from build123d import *

# Parameters (mm, degrees)
SKETCH1_W           = 20
SKETCH1_H           = 15
SKETCH1_W_2         = 15.2
SKETCH1_H_2         = 10.7
BOSS_EXTRUDE1_DEPTH = 21
SKETCH2_W           = 20
SKETCH2_H           = 15
SKETCH2_W_2         = 6.666666666
SKETCH2_H_2         = 5
BOSS_EXTRUDE2_DEPTH = 2
HOLE1_START         = -7.5
HOLE1_OUTLINE_R     = 1.25
HOLE1_DEPTH         = 15
FILLET1_R           = 1
SKETCH4_W           = 7
SKETCH4_H           = 3
CUT_EXTRUDE1_DEPTH  = 28.676705006


# Read off the part's stored shape, not the designer's step: Hole1
with BuildPart() as part:
    # Sketch1 → Boss-Extrude1 (new body)
    with BuildSketch(Plane(origin=(0, 0, 0), x_dir=(1, 0, 0), z_dir=(0, 1, 0))):
        Rectangle(SKETCH1_W, SKETCH1_H)
        Rectangle(SKETCH1_W_2, SKETCH1_H_2, mode=Mode.SUBTRACT)
    extrude(amount=BOSS_EXTRUDE1_DEPTH)

    # Sketch2 → Boss-Extrude2 (add)
    with BuildSketch(Plane.XZ):
        Rectangle(SKETCH2_W, SKETCH2_H)
        Rectangle(SKETCH2_W_2, SKETCH2_H_2, mode=Mode.SUBTRACT)
    extrude(amount=BOSS_EXTRUDE2_DEPTH)

    # Hole1 outline → Hole1 (cut)
    with BuildSketch(Plane.XY.offset(HOLE1_START)):
        with Locations((5.8, 3)):
            Circle(HOLE1_OUTLINE_R)
        with Locations((-5.8, 3)):
            Circle(HOLE1_OUTLINE_R)
    extrude(amount=HOLE1_DEPTH, mode=Mode.SUBTRACT)

    # Fillet1
    fillet1_edges = [part.edges().sort_by_distance(p)[0] for p in [
        (-10, 21, 0),
        (7.6, 21, 0),
        (0, 21, 7.5),
        (0, 21, -5.35),
        (-7.6, 21, 0),
        (0, 21, 5.35),
        (10, 21, 0),
        (10, 9.5, 7.5),
        (-10, 9.5, 7.5),
        (-10, 9.5, -7.5),
        (10, 9.5, -7.5),
        (0, 21, -7.5),
    ]]
    fillet(fillet1_edges, radius=FILLET1_R)

    # Sketch4 → Cut-Extrude1 (cut, through all)
    with BuildSketch(Plane.XY.offset(7.5)):
        with Locations((0.17, -0.5)):
            Rectangle(SKETCH4_W, SKETCH4_H)
    extrude(amount=-CUT_EXTRUDE1_DEPTH, mode=Mode.SUBTRACT)


solid = part.part
Design review of the part built by this model. Coordinates are the model's own, in mm. A direction names the side the tool comes from. Round coordinates to 2 decimals unless told otherwise and drop trailing zeros. Loops run counter-clockwise (first coordinate to the right, second up) from the corner with the lowest first, then second, coordinate; pieces in that order, holes last. Notation, with made-up numbers: M -12,-4.75 L 44,-4.75 A30 ccw 44,31.25 Z; hole C 68.25,-26.5 d4. An arc over 180 degrees is marked long. Answer as a JSON object with one key per item and string values.
Item 1: Machinability: for faces 4 (the cylindrical face through (-9.715, 9.154, 7.199)), 5 (the flat face through (0, 1, -6)), 6 (the flat face through (-5, 0, 0)), which of the approach directions +Z, -Z, +X, -X, +Y, -Y give a long, thin tool a straight path to every point of the face, cutting with its end or side? Answer none if there is none.
Answer sheet:
{"face 4": "+Z, -X, +Y, -Y", "face 5": "+Z, -Z, -Y", "face 6": "+Y"}
Item 2: We need section A-A on z = 1.5. Give the boundary of the cut face in (x, y), and give its area (3 significant figures).
Answer sheet:
{"outline": "M -10,-2 L -3.33,-2 L -3.33,0 L -7.6,0 L -7.6,20 A1 ccw -8.6,21 L -9,21 A1 ccw -10,20 Z; M 3.67,-2 L 10,-2 L 10,20 A1 ccw 9,21 L 8.6,21 A1 ccw 7.6,20 L 7.6,0 L 3.67,0 Z", "area": "126 mm^2"}
Item 3: Clearance check with flat-ended pins moving along their axes: P1, Ø1.1, axis at x = -1.5, z = -6, coming from the -Y side; P2, Ø2, axis at x = -5.8, y = 3, coming from the -Z side. State where each tip first meets the part, or that it passes through.
Answer sheet:
{"P1": "stops at y = 1", "P2": "passes through"}
Item 4: We need section B-B on x = 5.8. Give the boundary of the cut face in (y, z), and give its area (3 significant figures).
Answer sheet:
{"outline": "M -2,-7.5 L 1.75,-7.5 L 1.75,-5.35 L 0,-5.35 L 0,5.35 L 1.75,5.35 L 1.75,7.5 L -2,7.5 Z; M 4.25,-7.5 L 20,-7.5 A1 ccw 21,-6.5 L 21,-6.35 A1 ccw 20,-5.35 L 4.25,-5.35 Z; M 4.25,5.35 L 20,5.35 A1 ccw 21,6.35 L 21,6.5 A1 ccw 20,7.5 L 4.25,7.5 Z", "area": "109 mm^2"}
Item 5: We need section D-D on x = 2.25. Give the boundary of the cut face in (y, z), and give its area (3 significant figures).
Answer sheet:
{"outline": "M 1,-7.5 L 20,-7.5 A1 ccw 21,-6.5 L 21,-6.35 A1 ccw 20,-5.35 L 1,-5.35 Z; M 1,5.35 L 20,5.35 A1 ccw 21,6.35 L 21,6.5 A1 ccw 20,7.5 L 1,7.5 Z", "area": "85.1 mm^2"}
Item 6: We need section C-C on y = 10.25. Give the boundary of the cut face in (x, z).
Answer sheet:
{"outline": "M -10,-6.5 A1 ccw -9,-7.5 L 9,-7.5 A1 ccw 10,-6.5 L 10,6.5 A1 ccw 9,7.5 L -9,7.5 A1 ccw -10,6.5 Z; hole M -7.6,-5.35 L 7.6,-5.35 L 7.6,5.35 L -7.6,5.35 Z"}
Item 7: Wall thickness on L1, parallel to X at y = 3, z = 5.85; L2, parallel to Z at x = 7.5, y = 18.5; L3, parallel to X at y = 15, z = 0: over which ranges is each line inside the solid? List them lowest first. Write a range as from..to.
Answer sheet:
{"L1": "x = -10..-7.05, -4.55..4.55, 7.05..10", "L2": "z = -7.5..-5.35, 5.35..7.5", "L3": "x = -10..-7.6, 7.6..10"}
Item 8: The part is to be moulded in two halves that separate along Y. For faces 1 (the flat face through (3.67, -1, 0)), 2 (the cylindrical face through (-4.61, 3.38, -6.44)), 3 (the cylindrical face through (9.699, 20.715, -0.091)), say which applies: pulls with the +Y half, pulls with the -Y half, needs draft (parallel to the pull), parting line crosses it, or undercut.
Answer sheet:
{"face 1": "needs draft", "face 2": "undercut", "face 3": "pulls with the +Y half"}
